Autodesk Inventor part; units mm, degrees
ref_plane "YZ Plane" through (0, 0, 0) normal (1, 0, 0) x (0, 1, 0)
ref_plane "XZ Plane" through (0, 0, 0) normal (0, 1, 0) x (-1, 0, 0)
ref_plane "XY Plane" through (0, 0, 0) normal (0, 0, 1) x (1, 0, 0)
sketch "Sketch1" plane through (0, 0, 0) normal (0, 0, 1) x (1, 0, 0)
  line L0 (-43.7903, 41.0199) -> (46.7097, 41.0199)
  line L1 (46.7097, 41.0199) -> (46.7097, -19.9801)
  line L2 (46.7097, -19.9801) -> (-43.7903, -19.9801)
  line L3 (-43.7903, -19.9801) -> (-43.7903, 41.0199)
  point P0 (0, 0)
  dimension "d0" = 90.5
  dimension "d1" = 61
extrude "Extrusion1" add sketch "Sketch1" along normal blind 1.5
sketch "Sketch2" plane through (0, 0, 1.5) normal (0, 0, 1) x (1, 0, 0)
  line L0 (-42.7903, 39.5199) -> (45.2097, 39.5199)
  line L1 (45.2097, 39.5199) -> (45.2097, -18.4801)
  line L2 (45.2097, -18.4801) -> (-42.7903, -18.4801)
  line L3 (-42.7903, -18.4801) -> (-42.7903, 39.5199)
  line L4 (-43.7903, 41.0199) -> (46.7097, 41.0199)
  line L5 (46.7097, 41.0199) -> (46.7097, -19.9801)
  line L6 (46.7097, -19.9801) -> (-43.7903, -19.9801)
  line L7 (-43.7903, -19.9801) -> (-43.7903, 41.0199)
  point P0 (0, 0)
  dimension "d4" = 1.5
  dimension "d5" = 1.5
  dimension "d6" = 1.5
  dimension "d7" = 1
extrude "Extrusion2" add sketch "Sketch2" along normal blind 16
sketch "Sketch3" plane through (-43.7903, -19.9801, 0) normal (-1, 0, 0) x (0, 0, 1)
  line L0 (17.5, 1.5) -> (17.5, 59.5)
  line L1 (17.5, 20.5) -> (5.5, 20.5)
  line L2 (5.5, 20.5) -> (5.5, 3.5)
  line L3 (5.5, 3.5) -> (17.5, 3.5)
  line L4 (17.5, 3.5) -> (17.5, 20.5)
  line L5 (17.5, 38) -> (3.5, 38)
  line L6 (3.5, 38) -> (3.5, 24)
  line L7 (3.5, 24) -> (17.5, 24)
  line L8 (17.5, 24) -> (17.5, 38)
  line L9 (17.5, 56.5) -> (3.5, 56.5)
  line L10 (3.5, 56.5) -> (3.5, 42.5)
  line L11 (3.5, 42.5) -> (17.5, 42.5)
  line L12 (17.5, 42.5) -> (17.5, 56.5)
  line L13 (0, 0) -> (17.5, 0)
  point P0 (0, 19.9801)
  dimension "d10" = 3.5
  dimension "d11" = 12
  dimension "d12" = 17
  dimension "d13" = 3.5
  dimension "d14" = 14
  dimension "d15" = 14
  dimension "d16" = 14
  dimension "d17" = 4.5
  dimension "d18" = 14
extrude "Extrusion3" cut sketch "Sketch3" against normal blind 1
sketch "Sketch4" plane through (0, 0, 1.5) normal (0, 0, 1) x (1, 0, 0)
  line L0 (45.2097, 39.5199) -> (-15.7903, 39.5199)
  line L1 (-15.7903, 39.5199) -> (-15.7903, 30.5199)
  line L2 (-15.7903, 30.5199) -> (45.2097, 30.5199)
  line L3 (45.2097, 30.5199) -> (45.2097, 39.5199)
  point P0 (0, 0)
  dimension "d21" = 61
  dimension "d22" = 9
extrude "Extrusion4" cut sketch "Sketch4" against normal blind 1.5
sketch "Sketch5" plane through (0, 0, 1.5) normal (0, 0, 1) x (1, 0, 0)
  line L0 (45.2097, 30.5199) -> (-15.7903, 30.5199)
  line L1 (-15.7903, 30.5199) -> (-15.7903, 29.0199)
  line L2 (-15.7903, 29.0199) -> (45.2097, 29.0199)
  line L3 (45.2097, 29.0199) -> (45.2097, 30.5199)
  line L4 (-42.7903, 39.5199) -> (45.2097, 39.5199)
  line L5 (-15.7903, 29.0199) -> (-17.2903, 29.0199)
  line L6 (-17.2903, 29.0199) -> (-17.2903, 39.5199)
  line L7 (-17.2903, 39.5199) -> (-15.7903, 39.5199)
  line L8 (-15.7903, 39.5199) -> (-15.7903, 29.0199)
  line L9 (46.7097, 41.0199) -> (46.7097, -19.9801)
  line L10 (45.2097, -18.4801) -> (45.2097, 30.5199)
  point P0 (0, 0)
  dimension "d25" = 1.5
  dimension "d26" = 1.5
  dimension "d28" = 61
  dimension "d29" = 9
extrude "Extrusion5" add sketch "Sketch5" along normal blind 16
sketch "Sketch6" plane through (0, 0, 17.5) normal (0, 0, 1) x (1, 0, 0)
  line L0 (-43.7903, 0.5199) -> (-42.7903, 0.5199)
  line L1 (-42.7903, 4.0199) -> (-43.7903, 4.0199)
  line L2 (-42.7903, 0.5199) -> (-42.7903, 4.0199)
  line L3 (-43.7903, 4.0199) -> (-43.7903, 0.5199)
  line L4 (-43.7903, -19.9801) -> (-43.7903, 41.0199)
  line L5 (-43.2903, 4.0199) -> (-43.7903, 4.0199)
  line L6 (-43.7903, 4.0199) -> (-43.7903, 3.0199)
  line L7 (-43.7903, 3.0199) -> (-43.2903, 3.0199)
  line L8 (-43.2903, 3.0199) -> (-43.2903, 4.0199)
  point P0 (0, 0)
  dimension "d32" = 3.5
  dimension "d33" = 1
  dimension "d34" = 0.5
  dimension "d35" = 1
extrude "Extrusion6" cut sketch "Sketch6" against normal blind 12 contours L3 L1 L8 L7
sketch "Sketch7" plane through (0, 0, 17.5) normal (0, 0, 1) x (1, 0, 0)
  line L0 (-43.7903, 18.0199) -> (-42.7903, 18.0199)
  line L1 (-43.7903, 22.5199) -> (-43.7903, 18.0199)
  line L2 (-43.2903, 18.0199) -> (-43.7903, 18.0199)
  line L3 (-43.7903, 18.0199) -> (-43.7903, 19.0199)
  line L4 (-43.7903, 19.0199) -> (-43.2903, 19.0199)
  line L5 (-43.2903, 19.0199) -> (-43.2903, 18.0199)
  point P0 (0, 0)
  dimension "d38" = 1
extrude "Extrusion7" cut sketch "Sketch7" against normal blind 12
sketch "Sketch8" plane through (0, 0, 17.5) normal (0, 0, 1) x (1, 0, 0)
  line L0 (-43.7903, 22.5199) -> (-43.7903, 19.0199)
  line L1 (-43.2903, 22.5199) -> (-43.7903, 22.5199)
  line L2 (-43.7903, 22.5199) -> (-43.7903, 21.5199)
  line L3 (-43.7903, 21.5199) -> (-43.2903, 21.5199)
  line L4 (-43.2903, 21.5199) -> (-43.2903, 22.5199)
  line L5 (-42.7903, 22.5199) -> (-43.7903, 22.5199)
  point P0 (0, 0)
  dimension "d41" = 0.5
  dimension "d42" = 1
  dimension "d43" = 1
extrude "Extrusion8" cut sketch "Sketch8" against normal blind 12
sketch "Sketch9" plane through (0, 0, 17.5) normal (0, 0, 1) x (1, 0, 0)
  line L0 (-43.7903, 36.5199) -> (-42.7903, 36.5199)
  line L1 (-43.7903, 41.0199) -> (-43.7903, 36.5199)
  line L2 (-43.2903, 36.5199) -> (-43.7903, 36.5199)
  line L3 (-43.7903, 36.5199) -> (-43.7903, 37.5199)
  line L4 (-43.7903, 37.5199) -> (-43.2903, 37.5199)
  line L5 (-43.2903, 37.5199) -> (-43.2903, 36.5199)
  point P0 (0, 0)
  dimension "d46" = 1
  dimension "d47" = 0.5
extrude "Extrusion9" cut sketch "Sketch9" against normal blind 12
sketch "Sketch10" plane through (-43.7903, -19.9801, 0) normal (0, -1, 0) x (1, 0, 0)
  line L0 (29.5, 17.5) -> (37.5, 17.5)
  line L1 (37.5, 17.5) -> (37.5, 14)
  line L2 (37.5, 14) -> (29.5, 14)
  line L3 (29.5, 14) -> (29.5, 17.5)
  line L4 (0, 0) -> (0, 17.5)
  line L5 (47.5, 17.5) -> (63.5, 17.5)
  line L6 (63.5, 17.5) -> (63.5, 14)
  line L7 (63.5, 14) -> (47.5, 14)
  line L8 (47.5, 14) -> (47.5, 17.5)
  line L9 (90.5, 0) -> (90.5, 17.5)
  point P0 (43.7903, 0)
  dimension "d50" = 29.5
  dimension "d51" = 8
  dimension "d53" = 16
  dimension "d57" = 10
extrude "Extrusion10" cut sketch "Sketch10" against normal blind 1.5
sketch "Sketch11" plane through (-43.7903, -19.9801, 0) normal (0, -1, 0) x (1, 0, 0)
  line L0 (63.5, 17.5) -> (63.5, 14)
  line L1 (90.5, 0) -> (90.5, 17.5)
  line L2 (63.5, 16.6) -> (90.5, 16.6)
  line L3 (90.5, 16.6) -> (90.5, 15.5)
  line L4 (90.5, 15.5) -> (63.5, 15.5)
  line L5 (63.5, 15.5) -> (63.5, 16.6)
  line L6 (37.5, 17.5) -> (37.5, 14)
  line L7 (47.5, 14) -> (47.5, 17.5)
  line L8 (37.5, 16.6) -> (47.5, 16.6)
  line L9 (47.5, 16.6) -> (47.5, 15.5)
  line L10 (47.5, 15.5) -> (37.5, 15.5)
  line L11 (37.5, 15.5) -> (37.5, 16.6)
  line L12 (0, 0) -> (0, 17.5)
  line L13 (29.5, 14) -> (29.5, 17.5)
  line L14 (0, 16.6) -> (29.5, 16.6)
  line L15 (29.5, 16.6) -> (29.5, 15.5)
  line L16 (29.5, 15.5) -> (0, 15.5)
  line L17 (0, 15.5) -> (0, 16.6)
  line L18 (63.5, 17.5) -> (90.5, 17.5)
  line L19 (37.5, 17.5) -> (47.5, 17.5)
  line L20 (0, 17.5) -> (29.5, 17.5)
  point P0 (43.7903, 0)
  dimension "d61" = 1.1
  dimension "d62" = 0.9
  dimension "d63" = 1.1
  dimension "d64" = 0.9
  dimension "d65" = 1.1
  dimension "d66" = 0.9
extrude "Extrusion11" cut sketch "Sketch11" against normal blind 1 contours L2 L1 L4 L0 | L8 L7 L10 L6 | L12 L14 L13 L16
sketch "Sketch12" plane through (-43.7903, 41.0199, 0) normal (0, 1, 0) x (1, 0, 0)
  line L0 (90.5, 0) -> (90.5, -17.5)
  line L1 (0, 0) -> (0, -17.5)
  line L2 (90.5, -16.6) -> (0, -16.6)
  line L3 (0, -16.6) -> (0, -15.5)
  line L4 (0, -15.5) -> (90.5, -15.5)
  line L5 (90.5, -15.5) -> (90.5, -16.6)
  line L6 (90.5, -17.5) -> (0, -17.5)
  point P0 (43.7903, 0)
  dimension "d69" = 1.1
  dimension "d70" = 0.9
extrude "Extrusion12" cut sketch "Sketch12" against normal blind 1 contours L0 L2 L1 L4
sketch "Sketch13" plane through (0, 0, 17.5) normal (0, 0, 1) x (1, 0, 0)
  line L0 (-42.7903, -16.4801) -> (-43.7903, -16.4801)
  line L1 (-43.7903, -16.4801) -> (-43.7903, -19.9801)
  line L2 (-43.7903, -19.9801) -> (-42.7903, -19.9801)
  line L3 (-42.7903, -19.9801) -> (-42.7903, -16.4801)
  point P0 (0, 0)
extrude "Extrusion13" cut sketch "Sketch13" against normal blind 1
sketch "Sketch14" plane through (0, 0, 17.5) normal (0, 0, 1) x (1, 0, 0)
  line L0 (-42.7903, 4.0199) -> (-43.7903, 4.0199)
  line L1 (-43.7903, 4.0199) -> (-43.7903, 0.5199)
  line L2 (-43.7903, 0.5199) -> (-42.7903, 0.5199)
  line L3 (-42.7903, 0.5199) -> (-42.7903, 4.0199)
  point P0 (0, 0)
extrude "Extrusion14" cut sketch "Sketch14" against normal blind 1
sketch "Sketch15" plane through (0, 0, 17.5) normal (0, 0, 1) x (1, 0, 0)
  line L0 (-43.7903, 21.5199) -> (-43.7903, 19.0199)
  line L1 (-42.7903, 22.5199) -> (-43.7903, 22.5199)
  line L2 (-43.7903, 22.5199) -> (-43.7903, 20.2699)
  line L3 (-43.7903, 20.2699) -> (-42.7903, 20.2699)
  line L4 (-42.7903, 20.2699) -> (-42.7903, 22.5199)
  line L5 (-42.7903, 18.0199) -> (-43.7903, 18.0199)
  line L6 (-43.7903, 18.0199) -> (-43.7903, 20.2699)
  line L7 (-43.7903, 20.2699) -> (-42.7903, 20.2699)
  line L8 (-42.7903, 20.2699) -> (-42.7903, 18.0199)
  point P0 (0, 0)
extrude "Extrusion15" cut sketch "Sketch15" against normal blind 1
sketch "Sketch16" plane through (0, 0, 17.5) normal (0, 0, 1) x (1, 0, 0)
  line L0 (-43.7903, 41.0199) -> (-42.7903, 41.0199)
  line L1 (-42.7903, 41.0199) -> (-42.7903, 36.5199)
  line L2 (-42.7903, 36.5199) -> (-43.7903, 36.5199)
  line L3 (-43.7903, 36.5199) -> (-43.7903, 41.0199)
  point P0 (0, 0)
extrude "Extrusion16" cut sketch "Sketch16" against normal blind 1
sketch "Sketch17" plane through (0, 0, 17.5) normal (0, 0, 1) x (1, 0, 0)
  line L0 (46.7097, -19.9801) -> (45.0097, -19.9801)
  line L1 (45.0097, -19.9801) -> (45.0097, 41.0199)
  line L2 (45.0097, 41.0199) -> (46.7097, 41.0199)
  line L3 (46.7097, 41.0199) -> (46.7097, -19.9801)
  point P0 (0, 0)
  dimension "d81" = 61
  dimension "d84" = 1.7
extrude "Extrusion17" cut sketch "Sketch17" against normal blind 1
properties part number "raspi_enclosure2"
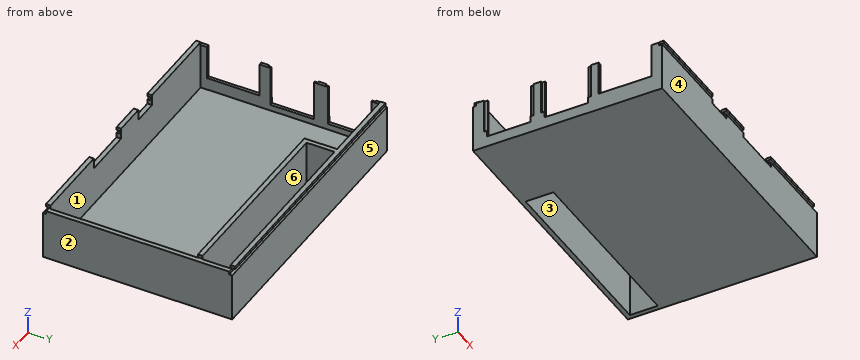
Model file for the job. Use its own axes, mm. Face numbers are marked on the shaded views. A direction names the side the tool comes from. Give positions to 0.01 mm unless a question says otherwise; leave off trailing zeros. Loops run counter-clockwise (first coordinate to the right, second up) from the corner with the lowest first, then second, coordinate; pieces in that order, holes last. Notation, with made-up numbers: (-32.5, 21) - (11.5, 21) arc R31 ccw to (11.5, 47) - close; hole circle Ø3 at (-2.5, 86). An arc over 180 degrees is marked (long way). Use one line per item in the form item = value.
(1) Cut at B-B (y = 32.5). Give the cut face in (x, z), then the cut area to 4 significant figures.
Determined:
outline = (-43.79, 0) - (-15.79, 0) - (-15.79, 17.5) - (-17.29, 17.5) - (-17.29, 1.5) - (-42.79, 1.5) - (-42.79, 3.5) - (-43.79, 3.5) - close; (45.21, 0) - (46.71, 0) - (46.71, 16.5) - (45.21, 16.5) - close
area = 92.75 mm^2
(2) Drop flat-ended pins along their axis: P1, Ø0.5, axis at y = 37, z = 10, coming from the -X side; P2, Ø2, axis at x = -30, y = 33.5, coming from the +Z side; P3, Ø0.8, axis at x = 13.5, y = -19, coming from the +Z side. Give the stop position or say it passes through.
Determined:
P1 = -43.29
P2 = 1.5
P3 = 14
(3) Cut at A-A (z = 7.75). Count the separate pieces of the cut face and the enclosed holes in it, then the cut area to 3 significant figures.
Determined:
separate_pieces = 3
enclosed_holes = 1
area = 477 mm^2
(4) Drill centre lines: L1, parallel to Y at x = 14, z = 3.75; L2, parallel to X at y = 35, z = 7.5; L3, parallel to X at y = 1, z = 13. Where is each one in solid material? Low to high.
Determined:
L1 = -19.98 to -18.48, 29.02 to 30.52, 39.52 to 41.02
L2 = -17.29 to -15.79, 45.21 to 46.71
L3 = -43.79 to -42.79, 45.21 to 46.71
(5) 3-axis set-ups, long thin cutter, end or side, ignore diameter. For the marked faces 1, 2 and 3: which of +Z, -Z, +X, -X, +Y, -Y reach the whole face in a straight line?
Determined:
face_1 = +Z
face_2 = +Z, -Z, +X, +Y, -Y
face_3 = +Z, -Z
(6) Cut at C-C (x = 21.5). Give the cut face in (y, z).
Determined:
outline = (-19.98, 0) - (30.52, 0) - (30.52, 17.5) - (29.02, 17.5) - (29.02, 1.5) - (-18.48, 1.5) - (-18.48, 17.5) - (-19.98, 17.5) - (-19.98, 16.6) - (-18.98, 16.6) - (-18.98, 15.5) - (-19.98, 15.5) - close; (39.52, 0) - (41.02, 0) - (41.02, 15.5) - (40.02, 15.5) - (40.02, 16.6) - (41.02, 16.6) - (41.02, 17.5) - (39.52, 17.5) - close
(7) Cut at D-D (x = -19). Give the cut face in (y, z), then the cut area to 3 significant figures.
Determined:
outline = (-19.98, 0) - (41.02, 0) - (41.02, 15.5) - (40.02, 15.5) - (40.02, 16.6) - (41.02, 16.6) - (41.02, 17.5) - (39.52, 17.5) - (39.52, 1.5) - (-18.48, 1.5) - (-18.48, 17.5) - (-19.98, 17.5) - (-19.98, 16.6) - (-18.98, 16.6) - (-18.98, 15.5) - (-19.98, 15.5) - close
area = 137 mm^2
(8) Pull direction Y, two halves, no side cores. Call the marked faces 4, 5 and 6: pulls with the +Y half, pulls with the -Y half, needs draft (parallel to the pull), parting line crosses it, or undercut.
Determined:
face_4 = pulls with the -Y half
face_5 = pulls with the +Y half
face_6 = undercut
